Here's how the part is built. I have some questions about the finished solid (model axes, mm). Face numbers are marked on the shaded views. A direction names the side the tool comes from. Give positions to 0.01 mm unless a question says otherwise; leave off trailing zeros. Loops run counter-clockwise (first coordinate to the right, second up) from the corner with the lowest first, then second, coordinate; pieces in that order, holes last. Notation, with made-up numbers: (48, -24) - (98, -24) arc R4 cw to (98, -18) - close; hole circle Ø1 at (85, -30). An arc over 180 degrees is marked (long way). Return JSON: item names as keys, results as strings. Group by question number.
(1) I need wall thicknesses on probe 1 along Y at (x, z) = (-32.5, -1.5); probe 2 along X at (y, z) = (170, 1); probe 3 along Y at (x, z) = (-37.5, -1.5). Which ranges of each line are inside material? Lowest first, please. Write a range as [from, to].
(2) For P1, Ø3, axis at y = 169.79, z = 0, coming from the -X side, with a flat end and sliding along its axis, tell me the tip position at first contact or that it passes through.
(3) If we section it at D-D (x = -55.5): Please give me the cut outline in (y, z) (3 decimals).
(4) On a 3-axis mill with a long thin cutter (end or side, diameter ignored), from which of +Z, -Z, +X, -X, +Y, -Y can I reach the whole of each face in a straight line? I mean the marked faces 1 and 2. Say none if no direction works.
(5) If we section it at B-B (y = 170.25): Please give me the cut outline in (x, z) (3 decimals).
(6) If we section it at A-A (x = -32.5): Please give me the cut outline in (y, z) (3 decimals), then the cut area to 3 significant figures.
(7) If we section it at C-C (z = -0.5): Please give me the cut outline in (x, y).
```python
from build123d import *

# Parameters (mm, degrees)
SKETCH1_R                = 2.15
BOSS_EXTRUDE1_DEPTH      = 3.175
BOSS_EXTRUDE1_DEPTH_BACK = 3.175
SKETCH2_R                = 1.35
CUT_EXTRUDE1_DEPTH       = 20.866025
SKETCH3_R                = 1.6
CUT_EXTRUDE2_DEPTH       = 5
FILLET1_R                = 0.3


with BuildPart() as part:
    # Sketch1 → Boss-Extrude1 (new body, two sides)
    with BuildSketch(Plane.XY) as boss_extrude1_sk:
        with BuildLine():
            Line((-9.5, 164.786291501), (-59.5, 164.786291501))
            Line((-59.5, 164.786291501), (-59.5, 184.786291501))
            Line((-59.5, 184.786291501), (-29.2, 184.786291501))
            Line((-29.2, 184.786291501), (-19.2, 174.786291501))
            ThreePointArc((-19.2, 174.786291501), (-17.7, 173.286291501), (-16.2, 174.786291501))
            Line((-16.2, 174.786291501), (-9.5, 181.486291501))
            Line((-9.5, 181.486291501), (-9.5, 164.786291501))
        make_face()
        with Locations((-52.5, 179.786291501)):
            Circle(SKETCH1_R, mode=Mode.SUBTRACT)
        with Locations((-37.5, 179.786291501)):
            Circle(SKETCH1_R, mode=Mode.SUBTRACT)
        with Locations((-32.5, 169.786291501)):
            Circle(SKETCH1_R, mode=Mode.SUBTRACT)
    extrude(amount=BOSS_EXTRUDE1_DEPTH)
    extrude(boss_extrude1_sk.sketch, amount=-BOSS_EXTRUDE1_DEPTH_BACK)

    # Sketch2 → Cut-Extrude1 (cut)
    with BuildSketch(Plane.ZY.offset(59.5)):
        with Locations((0, 169.786291501)):
            Circle(SKETCH2_R)
    extrude(amount=-CUT_EXTRUDE1_DEPTH, mode=Mode.SUBTRACT)

    # Sketch3 → Cut-Extrude2 (cut)
    with BuildSketch(Plane.ZY.offset(59.5)):
        with Locations((0, 169.786291501)):
            Circle(SKETCH3_R)
    extrude(amount=-CUT_EXTRUDE2_DEPTH, mode=Mode.SUBTRACT)

    # Fillet1
    fillet1_edges = [part.edges().sort_by_distance(p)[0] for p in [
        (-9.5, 181.486291501, 0),
    ]]
    fillet(fillet1_edges, radius=FILLET1_R)


solid = part.part
```
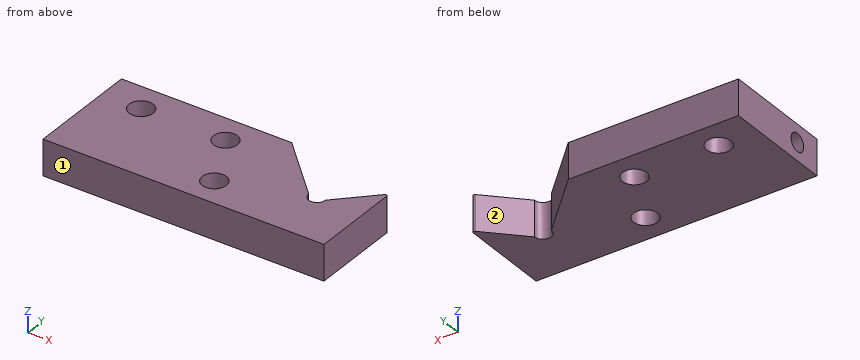
Values:
{
 "1": {"probe 1": "[164.79, 167.64], [171.94, 184.79]", "probe 2": "[-38.63, -34.64], [-30.36, -9.5]", "probe 3": "[164.79, 177.64], [181.94, 184.79]"},
 "2": {"P1": "x = -54.5"},
 "3": {"outline": "(164.786, -3.175) - (184.786, -3.175) - (184.786, 3.175) - (164.786, 3.175) - close; hole circle Ø3.2 at (169.786, 0)"},
 "4": {"face 1": "+Z, -Z, +X, -X, -Y", "face 2": "+Z, -Z, +Y"},
 "5": {"outline": "(-59.5, -3.175) - (-34.599, -3.175) - (-34.599, 3.175) - (-59.5, 3.175) - (-59.5, 1.531) - (-54.5, 1.531) - (-54.5, 1.268) - (-38.634, 1.268) - (-38.634, -1.268) - (-54.5, -1.268) - (-54.5, -1.531) - (-59.5, -1.531) - close; (-30.401, -3.175) - (-9.5, -3.175) - (-9.5, 3.175) - (-30.401, 3.175) - close"},
 "6": {"outline": "(164.786, -3.175) - (167.636, -3.175) - (167.636, 3.175) - (164.786, 3.175) - close; (171.936, -3.175) - (184.786, -3.175) - (184.786, 3.175) - (171.936, 3.175) - close", "area": "99.7 mm2"},
 "7": {"outline": "(-59.5, 164.79) - (-9.5, 164.79) - (-9.5, 180.76) arc R0.3 ccw to (-10.01, 180.97) - (-16.2, 174.79) arc R1.5 cw to (-19.2, 174.79) - (-29.2, 184.79) - (-59.5, 184.79) - (-59.5, 171.31) - (-54.5, 171.31) - (-54.5, 171.04) - (-38.63, 171.04) - (-38.63, 168.53) - (-54.5, 168.53) - (-54.5, 168.27) - (-59.5, 168.27) - close; hole circle Ø4.3 at (-52.5, 179.79); hole circle Ø4.3 at (-37.5, 179.79); hole circle Ø4.3 at (-32.5, 169.79)"}
}
